```python
from build123d import *

# Parameters (mm, degrees)
SZKIC1_W                                           = 596
SZKIC1_H                                           = 496
SZKIC1_R                                           = 45
SZKIC1_R_2                                         = 21
DODANIE_WYCI_GNI_CIE1_DEPTH                        = 36
SZKIC1_5_R                                         = 45
WYTNIJ_WYCI_GNI_CIE1_DEPTH                         = 4
POG_BIENIE_WALCOWE_POD_M16_WKR_T_Z_BEM_D           = 17.5
POG_BIENIE_WALCOWE_POD_M16_WKR_T_Z_BEM_CBORE_D     = 30.713
POG_BIENIE_WALCOWE_POD_M16_WKR_T_Z_BEM_CBORE_DEPTH = 21
SZKIC8_R                                           = 9
WYTNIJ_WYCI_GNI_CIE2_DEPTH                         = 777.05154468
SZKIC8_3_R                                         = 19
SZKIC8_3_R_2                                       = 9
WYTNIJ_WYCI_GNI_CIE3_DEPTH                         = 18
ZAOKR_GLENIE1_R                                    = 3
OTWORY_USTALAJ_CE_4_0MM1_D                         = 4
OTWORY_USTALAJ_CE_4_0MM1_DEPTH                     = 5
OTWORY_USTALAJ_CE_4_0MM1_TIP                       = 1.201721238
OTW_R_GWINTOWANY_M61_D                             = 5
OTW_R_GWINTOWANY_M61_DEPTH                         = 17
OTW_R_GWINTOWANY_M61_CSINK_D                       = 6.05
OTW_R_GWINTOWANY_M61_CSINK_ANGLE                   = 90
OTW_R_GWINTOWANY_M61_TIP                           = 1.502151548
OTW_R_GWINTOWANY_M161_D                            = 14
OTW_R_GWINTOWANY_M161_DEPTH                        = 42
OTW_R_GWINTOWANY_M161_CSINK_D                      = 16.05
OTW_R_GWINTOWANY_M161_CSINK_ANGLE                  = 90
OTW_R_GWINTOWANY_M161_TIP                          = 4.206024333


with BuildPart() as part:
    # Szkic1 → Dodanie-wyci_gni_cie1 (new body)
    # profile 1 of 2: a face of its own
    with BuildSketch(Plane(origin=(0, 0, 0), x_dir=(1, 0, 0), z_dir=(0, 1, 0))):
        with Locations((298, 248)):
            Rectangle(SZKIC1_W, SZKIC1_H)
        with Locations((298, 248)):
            Circle(SZKIC1_R, mode=Mode.SUBTRACT)
        with Locations(Location((560, 410, 0), (0, 0, 270))):
            Circle(SZKIC1_R_2, mode=Mode.SUBTRACT)
        with Locations(Location((36, 410, 0), (0, 0, 270))):
            Circle(SZKIC1_R_2, mode=Mode.SUBTRACT)
        with Locations(Location((560, 86, 0), (0, 0, 270))):
            Circle(SZKIC1_R_2, mode=Mode.SUBTRACT)
        with Locations(Location((36, 86, 0), (0, 0, 270))):
            Circle(SZKIC1_R_2, mode=Mode.SUBTRACT)
    # profile 2 of 2: a face of its own
    with BuildSketch(Plane(origin=(0, 0, 0), x_dir=(1, 0, 0), z_dir=(0, 1, 0))):
        with Locations((298, 248)):
            Circle(SZKIC1_R)
    extrude(amount=-DODANIE_WYCI_GNI_CIE1_DEPTH)

    # Szkic1_5 → Wytnij-wyci_gni_cie1 (cut)
    with BuildSketch(Plane(origin=(0, 0, 0), x_dir=(1, 0, 0), z_dir=(0, 1, 0))):
        with Locations(Location((298, 248, 0), (0, 0, 270))):
            Circle(SZKIC1_5_R)
    extrude(amount=-WYTNIJ_WYCI_GNI_CIE1_DEPTH, mode=Mode.SUBTRACT)

    # Pog_bienie walcowe pod M16 Wkr_t z _bem (through all)
    with Locations(Plane(origin=(83, 0, -410), x_dir=(0, 0, 1), z_dir=(0, 1, 0))):
        with Locations((0, 0), (0, 430), (324, 430), (324, 0)):
            CounterBoreHole(POG_BIENIE_WALCOWE_POD_M16_WKR_T_Z_BEM_D / 2, POG_BIENIE_WALCOWE_POD_M16_WKR_T_Z_BEM_CBORE_D / 2, POG_BIENIE_WALCOWE_POD_M16_WKR_T_Z_BEM_CBORE_DEPTH)

    # Szkic8 → Wytnij-wyci_gni_cie2 (cut, through all)
    with BuildSketch(Plane(origin=(0, -4, 0), x_dir=(1, 0, 0), z_dir=(0, 1, 0))):
        with Locations(Location((298, 248, 0), (0, 0, 270))):
            Circle(SZKIC8_R)
    extrude(amount=-WYTNIJ_WYCI_GNI_CIE2_DEPTH, mode=Mode.SUBTRACT)

    # Szkic8_3 → Wytnij-wyci_gni_cie3 (cut)
    with BuildSketch(Plane(origin=(0, -4, 0), x_dir=(1, 0, 0), z_dir=(0, 1, 0))):
        with Locations(Location((298, 248, 0), (0, 0, 270))):
            Circle(SZKIC8_3_R)
        with Locations(Location((298, 248, 0), (0, 0, 270))):
            Circle(SZKIC8_3_R_2, mode=Mode.SUBTRACT)
    extrude(amount=-WYTNIJ_WYCI_GNI_CIE3_DEPTH, mode=Mode.SUBTRACT)

    # Zaokr_glenie1
    zaokr_glenie1_edges = [part.edges().sort_by_distance(p)[0] for p in [
        (298, -22, -257),
    ]]
    fillet(zaokr_glenie1_edges, radius=ZAOKR_GLENIE1_R)

    # Otwory ustalaj_ce _4.0mm1
    with Locations(Plane(origin=(313, -22, -248), x_dir=(0, 0, 1), z_dir=(0, 1, 0))):
        with Locations((0, 0)):
            Hole(OTWORY_USTALAJ_CE_4_0MM1_D / 2, depth=OTWORY_USTALAJ_CE_4_0MM1_DEPTH)
            with Locations((0, 0, -(OTWORY_USTALAJ_CE_4_0MM1_DEPTH + OTWORY_USTALAJ_CE_4_0MM1_TIP / 2))):  # 118° drill point
                Cone(0, OTWORY_USTALAJ_CE_4_0MM1_D / 2, OTWORY_USTALAJ_CE_4_0MM1_TIP, mode=Mode.SUBTRACT)

    # Otw_r gwintowany M61
    with Locations(Plane(origin=(243, 0, -248), x_dir=(0, 0, 1), z_dir=(0, 1, 0))):
        with Locations((0, 0), (-55, 55), (0, 110), (55, 55)):
            CounterSinkHole(OTW_R_GWINTOWANY_M61_D / 2, OTW_R_GWINTOWANY_M61_CSINK_D / 2, depth=OTW_R_GWINTOWANY_M61_DEPTH, counter_sink_angle=OTW_R_GWINTOWANY_M61_CSINK_ANGLE)
            with Locations((0, 0, -(OTW_R_GWINTOWANY_M61_DEPTH + OTW_R_GWINTOWANY_M61_TIP / 2))):  # 118° drill point
                Cone(0, OTW_R_GWINTOWANY_M61_D / 2, OTW_R_GWINTOWANY_M61_TIP, mode=Mode.SUBTRACT)

    # Otw_r gwintowany M161
    with Locations(Plane(origin=(83, -18, 0), x_dir=(1, 0, 0), z_dir=(0, 0, 1))):
        with Locations((0, 0), (430, 0)):
            CounterSinkHole(OTW_R_GWINTOWANY_M161_D / 2, OTW_R_GWINTOWANY_M161_CSINK_D / 2, depth=OTW_R_GWINTOWANY_M161_DEPTH, counter_sink_angle=OTW_R_GWINTOWANY_M161_CSINK_ANGLE)
            with Locations((0, 0, -(OTW_R_GWINTOWANY_M161_DEPTH + OTW_R_GWINTOWANY_M161_TIP / 2))):  # 118° drill point
                Cone(0, OTW_R_GWINTOWANY_M161_D / 2, OTW_R_GWINTOWANY_M161_TIP, mode=Mode.SUBTRACT)


solid = part.part
```
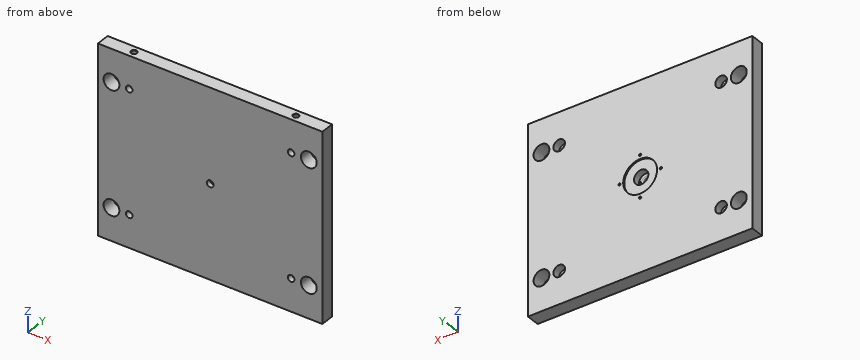
Read the model definition and answer for the solid it produces. Units are mm, in the model's axes. Give positions to 0.01 mm unless a question says otherwise; leave off trailing zeros. Loops run counter-clockwise (first coordinate to the right, second up) from the corner with the lowest first, then second, coordinate; pieces in that order, holes last.
Item 1: Each of these flat-tipped pins is pushed along its axis until it touches: pin 1 Ø15.5 at (x, z) = (509.5, -88.5) entering from +Y; pin 2 Ø16 at (x, z) = (513, -86) entering from +Y; pin 3 Ø4 at (x, z) = (353, -248) entering from +Y. Where does it stop, or does it pass through?
Item 2: Find the intervals of material crossed by line 1 along Z through (x, y) = (513, -29.25); line 2 along X through (y, z) = (-9, -248); line 3 along X through (y, z) = (-32, -410), in increasing order.
Item 3: The part is cut by section B-B (x = 36). Write down the section's boundary in (y, z), and give its area (3 significant figures).
Item 4: The part is cut by section A-A (z = -86). Write down the section's boundary in (x, y).
Taken from the geometry:
1. pin 1: stops at y = -21
1. pin 2: passes through
1. pin 3: stops at y = -17.3
2. line 1: z = -496 to -418.75, -401.25 to -94.75, -77.25 to 0
2. line 2: x = 0 to 240.5, 245.5 to 279, 317 to 350.5, 355.5 to 596
2. line 3: x = 0 to 15, 57 to 74.25, 91.75 to 504.25, 521.75 to 539, 581 to 596
3. outline: (-36, -496) - (0, -496) - (0, -431) - (-36, -431) - close; (-36, -389) - (0, -389) - (0, -107) - (-36, -107) - close; (-36, -65) - (0, -65) - (0, 0) - (-36, 0) - close
3. area: 14,800 mm2
4. outline: (0, -36) - (15, -36) - (15, 0) - (0, 0) - close; (57, -36) - (74.25, -36) - (74.25, -21) - (67.64, -21) - (67.64, 0) - (57, 0) - close; (91.75, -36) - (504.25, -36) - (504.25, -21) - (497.64, -21) - (497.64, 0) - (98.36, 0) - (98.36, -21) - (91.75, -21) - close; (521.75, -36) - (539, -36) - (539, 0) - (528.36, 0) - (528.36, -21) - (521.75, -21) - close; (581, -36) - (596, -36) - (596, 0) - (581, 0) - close
